```python
from build123d import *

# Parameters (mm, degrees)
FILLET1_R           = 1
BOSS_EXTRUDE1_DEPTH = 10
SKETCH4_R           = 1
BOSS_EXTRUDE2_DEPTH = 10


with BuildPart() as part:
    # Sketch2 → Revolve1 (revolve)
    with BuildSketch(Plane.XY):
        Polygon((0, 0), (0, 2), (8, 2), (8, 3), (10, 3), (10, 6.5), (21, 6.5), (21, 2), (23, 2), (23, 3), (25, 3), (25, 2), (31, 2), (31, 0), align=None)
    revolve(axis=Axis((31, 0, 0), (-1, 0, 0)))

    # Fillet1
    fillet1_edges = [part.edges().sort_by_distance(p)[0] for p in [
        (23, -2, 0),
        (21, -2, 0),
    ]]
    fillet(fillet1_edges, radius=FILLET1_R - 0.0001)  # a hair under: the kernel refuses the full size

    # Sketch3 → Boss-Extrude1 (add)
    with BuildSketch(Plane(origin=(0, 0, 0), x_dir=(1, 0, 0), z_dir=(0, 1, 0))):
        Polygon((16.75, 2.165063509), (14.25, 2.165063509), (13, 0), (14.25, -2.165063509), (16.75, -2.165063509), (18, 0), align=None)
    extrude(amount=BOSS_EXTRUDE1_DEPTH)

    # Sketch4 → Boss-Extrude2 (add)
    with BuildSketch(Plane(origin=(0, 10, 0), x_dir=(1, 0, 0), z_dir=(0, 1, 0))):
        with Locations(Location((15.5, 0, 0), (0, 0, 270))):
            Circle(SKETCH4_R)
    extrude(amount=BOSS_EXTRUDE2_DEPTH)


solid = part.part
```
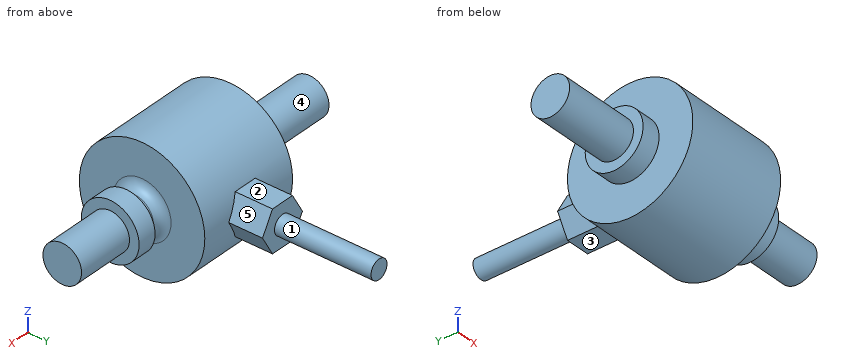
Could you check a few things on this model? Use its own coordinates, in mm. Face numbers are marked on the shaded views. A direction names the side the tool comes from. Coordinates: 2 decimals unless noted, no trailing zeros. Order: outer loops, then holes, each group sorted by start corner. A loop starts at its lowest first (then second) coordinate and runs counter-clockwise, first axis right, second up. Notation, with made-up numbers: M -2.75,69.5 L 13.25,69.5 A17 ccw 13.25,94.5 Z; hole C 46.25,81 d7. An arc over 180 degrees is marked long. Use one line per item in the form item = value. Start each with the question number.
1. For pin 1 (4 mm diameter, centred on x = 10.5, z = 5, fed in from -Y); pin 2 (3 mm diameter, centred on y = 7, z = 1, fed in from -X); pin 3 (4 mm diameter, centred on y = 12.5, z = -4, fed in from +X); pin 4 (1.2 mm diameter, centred on x = 15, y = 8.5, fed in from +Z), each with a flat end and sliding along its axis, tell me the tip position at first contact or that it passes through.
2. On a 3-axis mill with a long thin cutter (end or side, diameter ignored), from which of +Z, -Z, +X, -X, +Y, -Y can I reach the whole of each face in a straight line? I mean the marked faces 1, 2, 3, 4 and 5. Say none if no direction works.
3. Suppose I cut it at C-C on z = -4.25. Write out the boundary of the cut face in (x, y).
4. Suppose I cut it at B-B on x = 15.5. Write out the boundary of the cut face in (y, z).
5. Please list where these lines run through material, in increasing order: line 1 (X direction, y = -3, z = 3.25); line 2 (Z direction, x = 14.5, y = -4.25); line 3 (Y direction, x = 15, z = 1.25).
6. Suppose I cut it at D-D on x = 7. Write out the boundary of the cut face in (y, z), then the cut area to 3 significant figures.
Geometry says:
q1.pin_1 = -5.77
q1.pin_2 = 10
q1.pin_3 = through
q1.pin_4 = 2.17
q2.face_1 = +Y
q2.face_2 = +Z, +X, -X, +Y
q2.face_3 = -Z, +X, -X, +Y
q2.face_4 = -X
q2.face_5 = +Z, +X, +Y
q3.outline = M 10,-4.92 L 21,-4.92 L 21,4.92 L 10,4.92 Z
q4.outline = M 6.13,-2.17 L 10,-2.17 L 10,-1 L 20,-1 L 20,1 L 10,1 L 10,2.17 L 6.13,2.17 A6.5 ccw long Z
q5.line_1 = 10 to 21
q5.line_2 = -4.92 to 4.92
q5.line_3 = -6.38 to 10
q6.outline = C 0,0 d4
q6.area = 12.6 mm^2
